The model under review builds one solid part; all positions refer to its coordinate system, in mm. A direction names the side the tool comes from. Round coordinates to 2 decimals unless told otherwise and drop trailing zeros. Write each loop counter-clockwise with the first axis right and the second up, starting at its lowest first coordinate (ties: lowest second). Pieces come first, ordered by that corner, then holes.
Item 1: Machinability: for faces 4 (the face through (0, 8, 13)), 5 (the face through (-2.61, 12.73, 3.46)), 6 (the face through (25, 0, 10)), which of the approach directions +Z, -Z, +X, -X, +Y, -Y give a long, thin tool a straight path to every point of the face, cutting with its end or side? Answer none if there is none.
Item 2: Draft analysis for pull direction X (two halves, no side actions). For faces 1 (the face through (-2.8, -9.7, 0.3)), 2 (the face through (27.47, -0.04, 11.25)), 3 (the face through (-27, 0, 2)), state which applies: +X half, -X half, draft (parallel to the pull), parting line (faces both ways), or undercut.
Item 3: Clearance check with flat-ended pins moving along their axes: pin 1 Ø3 at (x, y) = (0, 11.25) entering from -Z; pin 2 Ø1.5 at (x, y) = (16.5, -6.5) entering from +Z; pin 3 Ø1.5 at (x, y) = (1, -12.5) entering from -Z; pin 4 Ø5 at (y, z) = (-9, 2) entering from -X. State where each tip first meets the part, or that it passes through.
Item 4: To check wall thickness, follow L1, parallel to Y at x = -0.5, z = 4.75; L2, parallel to Y at x = 0, z = 8.85. State the ranges of each line that lie inside material, in increasing order.
Item 5: Add section B-B (x = 0). State how many separate pieces and enclosed holes the cut face has, plus the area to 3 significant figures.
Item 6: Add section A-A (y = 15.5). Give the boundary of the cut face in (x, z), plus the area to 3 significant figures.
```python
from build123d import *

# Parameters (mm, degrees)
SKETCH1_W               = 60
SKETCH1_H               = 35
BOSS_EXTRUDE1_DEPTH     = 13
CUT_EXTRUDE1_DEPTH      = 64.837684937
CUT_EXTRUDE1_DEPTH_BACK = 64.837684937
SKETCH3_R               = 1.75
SKETCH5_R               = 1.75
CUT_EXTRUDE3_DEPTH      = 38.08436341
CHAMFER1_SIZE           = 5
CUT_EXTRUDE4_DEPTH      = 7
SKETCH4_W               = 60
SKETCH4_H               = 2.9
BOSS_EXTRUDE2_DEPTH     = 0.9
CHAMFER2_SIZE           = 0.5


with BuildPart() as part:
    # Sketch1 → Boss-Extrude1 (new body)
    with BuildSketch(Plane.XY):
        Rectangle(SKETCH1_W, SKETCH1_H)
    extrude(amount=BOSS_EXTRUDE1_DEPTH)

    # Sketch2 → Cut-Revolve1 (revolve, cut)
    with BuildSketch(Plane.XY.offset(13)):
        with BuildLine():
            Line((-25, 0), (-25, 8.218127455))
            ThreePointArc((-25, 8.218127455), (-24.486963528, 9.469250598), (-23.243251097, 10))
            ThreePointArc((-23.243251097, 10), (-15.040879193, 9.611248064), (-6.94833646, 8.218127455))
            ThreePointArc((-6.94833646, 8.218127455), (0, 7.408356031), (6.94833646, 8.218127455))
            ThreePointArc((6.94833646, 8.218127455), (15.040879193, 9.611248064), (23.243251097, 10))
            ThreePointArc((23.243251097, 10), (24.486963528, 9.469250598), (25, 8.218127455))
            Line((25, 8.218127455), (25, 0))
            Line((25, 0), (-25, 0))
        make_face()
    revolve(axis=Axis((25, 0, 13), (-1, 0, 0)), mode=Mode.SUBTRACT)

    # Sketch3 → Cut-Extrude1 (cut, two sides: drawn at the far end of the back side and taken through both)
    with BuildSketch(Plane(origin=(30, 0, 0), x_dir=(0, 0, -1), z_dir=(1, 0, 0)).offset(-CUT_EXTRUDE1_DEPTH_BACK)):
        with Locations((-13, 0)):
            Circle(SKETCH3_R)
    extrude(amount=CUT_EXTRUDE1_DEPTH + CUT_EXTRUDE1_DEPTH_BACK, mode=Mode.SUBTRACT)

    # Sketch5 → Cut-Extrude3 (cut, through all)
    with BuildSketch(Plane.XY.offset(13)):
        with Locations((0, 11.25)):
            Circle(SKETCH5_R)
        with Locations((0, -11.25)):
            Circle(SKETCH5_R)
    extrude(amount=-CUT_EXTRUDE3_DEPTH, mode=Mode.SUBTRACT)

    # Chamfer1
    chamfer1_edges = [part.edges().sort_by_distance(p)[0] for p in [
        (-30, 0, 0),
        (30, 0, 0),
    ]]
    chamfer(chamfer1_edges, length=CHAMFER1_SIZE)

    # Sketch6 → Cut-Extrude4 (cut)
    with BuildSketch(Plane(origin=(0, 0, 0), x_dir=(-1, 0, 0), z_dir=(0, 0, -1))):
        Polygon((3.464101615, 11.25), (1.732050808, 14.25), (-1.732050808, 14.25), (-3.464101615, 11.25), (-1.732050808, 8.25), (1.732050808, 8.25), align=None)
        Polygon((3.464101615, -11.25), (1.732050808, -8.25), (-1.732050808, -8.25), (-3.464101615, -11.25), (-1.732050808, -14.25), (1.732050808, -14.25), align=None)
    extrude(amount=-CUT_EXTRUDE4_DEPTH, mode=Mode.SUBTRACT)

    # Sketch4 → Boss-Extrude2 (add)
    with BuildSketch(Plane.XY.offset(13)):
        with Locations((0, 16.05)):
            Rectangle(SKETCH4_W, SKETCH4_H)
        with Locations((0, -16.05)):
            Rectangle(SKETCH4_W, SKETCH4_H)
    extrude(amount=BOSS_EXTRUDE2_DEPTH)

    # Chamfer2
    chamfer2_edges = [part.edges().sort_by_distance(p)[0] for p in [
        (-2.598076211, 9.75, 0),
        (-2.598076211, 12.75, 0),
        (0, 14.25, 0),
        (2.598076211, 12.75, 0),
        (2.598076211, 9.75, 0),
        (0, 8.25, 0),
        (-2.598076211, 9.75, 7),
        (0, 8.25, 7),
        (2.598076211, 9.75, 7),
        (2.598076211, 12.75, 7),
        (0, 14.25, 7),
        (-2.598076211, 12.75, 7),
        (-1.75, 11.25, 7),
        (-2.598076211, -12.75, 0),
        (-2.598076211, -9.75, 0),
        (0, -8.25, 0),
        (2.598076211, -9.75, 0),
        (2.598076211, -12.75, 0),
        (0, -14.25, 0),
        (-2.598076211, -12.75, 7),
        (0, -14.25, 7),
        (2.598076211, -12.75, 7),
        (2.598076211, -9.75, 7),
        (0, -8.25, 7),
        (-2.598076211, -9.75, 7),
        (-1.75, -11.25, 7),
    ]]
    chamfer(chamfer2_edges, length=CHAMFER2_SIZE)


solid = part.part
```
Numbers:
1. face 4: +Z, +X, -X
1. face 5: -Z
1. face 6: +Z
2. face 1: undercut
2. face 2: draft
2. face 3: -X half
3. pin 1: passes through
3. pin 2: stops at z = 6.48
3. pin 3: stops at z = 7
3. pin 4: stops at x = -29.5
4. L1: y = -17.5 to -14.25, -8.25 to 8.25, 14.25 to 17.5
4. L2: y = -17.5 to -13, -9.5 to -6.14, 6.14 to 9.5, 13 to 17.5
5. separate pieces: 3
5. enclosed holes: 0
5. area: 248 mm2
6. outline: (-30, 5) - (-25, 0) - (25, 0) - (30, 5) - (30, 13.9) - (-30, 13.9) - close
6. area: 809 mm2
